The listing builds one solid part. Answer for the finished solid, in the listing's coordinates (mm). A direction names the side the tool comes from. Coordinates: 2 decimals unless noted, no trailing zeros. Loops run counter-clockwise (first coordinate to the right, second up) from the corner with the lowest first, then second, coordinate; pieces in that order, holes last. Notation, with made-up numbers: (71.5, 33) - (95.5, 33) arc R19 cw to (95.5, 52) - close; hole circle Ø7 at (-5, 50). An arc over 180 degrees is marked (long way). Write each question's results on one line, items separated by ' | '. Start each with the question number.
(1) Determine the mould class of faces 1 (the flat face through (-1.3, 28, 1.3)), 2 (the flat face through (-1.12, 30.36, 0.64)), 3 (the cylindrical face through (0.9, 29.48, 2.86)) for opening direction Z: released by +Z, released by -Z, zero draft, split by the parting line, or undercut.
(2) Find section D-D on x = -2.5. Determine the outline of the cut face in (y, z), then the cut area to 3 significant figures.
(3) Consider line 1 (Y direction, x = 2.7, z = -0.5); line 2 (Y direction, x = 0.1, z = -1.2); line 3 (X direction, y = 13, z = 0.2). Determine where each line is inside the solid, lowest interval first. Write a range as from..to.
(4) Find section B-B on y = 12. Determine the outline of the cut face in (x, z).
(5) Find section A-A on x = 0. Determine the outline of the cut face in (y, z).
(6) Given pin 1 Ø3 at (y, z) = (13, -0.5) entering from +X; pin 2 Ø2 at (x, z) = (-0.5, 0) entering from +Y; pin 3 Ø3 at (x, y) = (-1, 16) entering from -Z; pin 4 Ø1.5 at (y, z) = (11, -1) entering from -X, each flat-ended and moving along its own axis, determine where each tip first touches the part or whether it passes through.
(7) For faces 4 (the flat face through (0, 0, 0)), 5 (the cylindrical face through (0.45, 13.8, 1.43)), 6 (the flat face through (1.12, 30.36, -0.64)), determine the directions among +Z, -Z, +X, -X, +Y, -Y from which every point of the face is accessible in a straight line to the end or side of a thin tool.
(8) Find section C-C on z = 1.95. Determine the outline of the cut face in (x, y), then the cut area to 3 significant figures.
from build123d import *

# Parameters (mm, degrees)
SKETCH1_R           = 1.5
SCREWSHAFT_DEPTH    = 28
SKETCH2_R           = 3
BOSS_EXTRUDE2_DEPTH = 3
CUT_EXTRUDE1_DEPTH  = 1.3


with BuildPart() as part:
    # Sketch1 → ScrewShaft (new body)
    with BuildSketch(Plane(origin=(0, 0, 0), x_dir=(1, 0, 0), z_dir=(0, 1, 0))):
        with Locations(Location((0, 0, 0), (0, 0, 270))):
            Circle(SKETCH1_R)
    extrude(amount=SCREWSHAFT_DEPTH)

    # Sketch2 → Boss-Extrude2 (add)
    with BuildSketch(Plane(origin=(0, 28, 0), x_dir=(1, 0, 0), z_dir=(0, 1, 0))):
        with Locations(Location((0, 0, 0), (0, 0, 270))):
            Circle(SKETCH2_R)
    extrude(amount=BOSS_EXTRUDE2_DEPTH)

    # Sketch3 → Cut-Extrude1 (cut)
    with BuildSketch(Plane(origin=(0, 31, 0), x_dir=(1, 0, 0), z_dir=(0, 1, 0))):
        Polygon((1.489563695, 0), (0.744781847, 1.29), (-0.744781847, 1.29), (-1.489563695, 0), (-0.744781847, -1.29), (0.744781847, -1.29), align=None)
    extrude(amount=-CUT_EXTRUDE1_DEPTH, mode=Mode.SUBTRACT)


solid = part.part
Values:
1) face 1: zero draft | face 2: undercut | face 3: split by the parting line
2) outline: (28, -1.66) - (31, -1.66) - (31, 1.66) - (28, 1.66) - close | area: 9.95 mm²
3) line 1: y = 28..31 | line 2: y = 0..29.7 | line 3: x = -1.49..1.49
4) outline: circle Ø3 at (0, 0)
5) outline: (0, -1.5) - (28, -1.5) - (28, -3) - (31, -3) - (31, -1.29) - (29.7, -1.29) - (29.7, 1.29) - (31, 1.29) - (31, 3) - (28, 3) - (28, 1.5) - (0, 1.5) - close
6) pin 1: stops at x = 1.5 | pin 2: stops at y = 31 | pin 3: stops at z = -1.5 | pin 4: stops at x = -1.48
7) face 4: +Z, -Z, +X, -X, -Y | face 5: -Y | face 6: +Y
8) outline: (-2.28, 28) - (2.28, 28) - (2.28, 31) - (-2.28, 31) - close | area: 13.7 mm²
